from build123d import *

# Parameters (mm, degrees)
BOSS_EXTRUDE1_DEPTH = 25
FILLET1_R           = 5
SHELL1_T            = -2
SKETCH2_R           = 6.175
CUT_EXTRUDE2_DEPTH  = 25
CUT_EXTRUDE4_DEPTH  = 25
SKETCH4_R           = 1.25
SKETCH4_R_2         = 0.5
BOSS_EXTRUDE2_DEPTH = 7
SKETCH5_W           = 50.970389208
SKETCH5_H           = 16.037024898
CUT_EXTRUDE5_DEPTH  = 1.5


with BuildPart() as part:
    # Sketch1 → Boss-Extrude1 (new body)
    with BuildSketch(Plane.XY):
        with BuildLine():
            Line((-50, -62.5), (50, -62.5))
            ThreePointArc((50, -62.5), (53.535533906, -61.035533906), (55, -57.5))
            Line((55, -57.5), (55, 57.5))
            ThreePointArc((55, 57.5), (53.535533906, 61.035533906), (50, 62.5))
            Line((50, 62.5), (-50, 62.5))
            ThreePointArc((-50, 62.5), (-53.535533906, 61.035533906), (-55, 57.5))
            Line((-55, 57.5), (-55, -57.5))
            ThreePointArc((-55, -57.5), (-53.535533906, -61.035533906), (-50, -62.5))
        make_face()
    extrude(amount=BOSS_EXTRUDE1_DEPTH)

    # Fillet1
    fillet1_edges = [part.edges().sort_by_distance(p)[0] for p in [
        (53.535533906, -61.035533906, 25),
        (55, 0, 25),
        (53.535533906, 61.035533906, 25),
        (0, 62.5, 25),
        (-53.535533906, 61.035533906, 25),
        (-55, 0, 25),
        (-53.535533906, -61.035533906, 25),
        (0, -62.5, 25),
    ]]
    fillet(fillet1_edges, radius=FILLET1_R)

    # Shell1
    shell1_openings = [part.faces().sort_by_distance(p)[0] for p in [
        (0, 0, 0),
    ]]
    offset(amount=SHELL1_T, openings=shell1_openings, kind=Kind.INTERSECTION)

    # Sketch2 → Cut-Extrude2 (cut)
    with BuildSketch(Plane.XY.offset(25)):
        with Locations((-37.5, -45)):
            Circle(SKETCH2_R)
        with Locations((-12.5, -45)):
            Circle(SKETCH2_R)
        with Locations((12.5, -45)):
            Circle(SKETCH2_R)
        with Locations((37.5, -45)):
            Circle(SKETCH2_R)
        with Locations((-37.5, -23)):
            Circle(SKETCH2_R)
        with Locations((-12.5, -23)):
            Circle(SKETCH2_R)
        with Locations((12.5, -23)):
            Circle(SKETCH2_R)
        with Locations((37.5, -23)):
            Circle(SKETCH2_R)
        with Locations((-37.5, -1)):
            Circle(SKETCH2_R)
        with Locations((-12.5, -1)):
            Circle(SKETCH2_R)
        with Locations((12.5, -1)):
            Circle(SKETCH2_R)
        with Locations((37.5, -1)):
            Circle(SKETCH2_R)
        with Locations((-37.5, 21)):
            Circle(SKETCH2_R)
        with Locations((-12.5, 21)):
            Circle(SKETCH2_R)
        with Locations((12.5, 21)):
            Circle(SKETCH2_R)
        with Locations((37.5, 21)):
            Circle(SKETCH2_R)
    extrude(amount=-CUT_EXTRUDE2_DEPTH, mode=Mode.SUBTRACT)

    # Sketch3 → Cut-Extrude4 (cut)
    with BuildSketch(Plane.ZY.offset(55)):
        with BuildLine():
            Line((14.181299903, 43.9), (16.681299903, 42.5))
            ThreePointArc((16.681299903, 42.5), (17.034853293, 42.646446609), (17.181299903, 43))
            Line((17.181299903, 43), (17.181299903, 50))
            ThreePointArc((17.181299903, 50), (17.034853293, 50.353553391), (16.681299903, 50.5))
            Line((16.681299903, 50.5), (14.181299903, 49.1))
            Line((14.181299903, 49.1), (14.181299903, 43.9))
        make_face()
    extrude(amount=-CUT_EXTRUDE4_DEPTH, mode=Mode.SUBTRACT)

    # Sketch4 → Boss-Extrude2 (add)
    # profile 1 of 4: a face of its own
    with BuildSketch(Plane(origin=(0, 0, 17.181299903), x_dir=(-1, 0, 0), z_dir=(0, 0, -1))):
        with Locations((50.75, 40.469217889)):
            Circle(SKETCH4_R)
        with Locations((50.75, 40.469217889)):
            Circle(SKETCH4_R_2, mode=Mode.SUBTRACT)
    # profile 2 of 4: a face of its own
    with BuildSketch(Plane(origin=(0, 0, 17.181299903), x_dir=(-1, 0, 0), z_dir=(0, 0, -1))):
        with Locations((50.75, 52.469217889)):
            Circle(SKETCH4_R)
        with Locations((50.75, 52.469217889)):
            Circle(SKETCH4_R_2, mode=Mode.SUBTRACT)
    # profile 3 of 4: a face of its own
    with BuildSketch(Plane(origin=(0, 0, 17.181299903), x_dir=(-1, 0, 0), z_dir=(0, 0, -1))):
        with Locations((4.25, 52.469217889)):
            Circle(SKETCH4_R)
        with Locations((4.25, 52.469217889)):
            Circle(SKETCH4_R_2, mode=Mode.SUBTRACT)
    # profile 4 of 4: a face of its own
    with BuildSketch(Plane(origin=(0, 0, 17.181299903), x_dir=(-1, 0, 0), z_dir=(0, 0, -1))):
        with Locations((4.25, 40.469217889)):
            Circle(SKETCH4_R)
        with Locations((4.25, 40.469217889)):
            Circle(SKETCH4_R_2, mode=Mode.SUBTRACT)
    extrude(amount=-BOSS_EXTRUDE2_DEPTH)

    # Sketch5 → Cut-Extrude5 (cut)
    with BuildSketch(Plane(origin=(0, 0, 17.181299903), x_dir=(-1, 0, 0), z_dir=(0, 0, -1))):
        with Locations((26.773560326, 46.339549131)):
            Rectangle(SKETCH5_W, SKETCH5_H)
    extrude(amount=-CUT_EXTRUDE5_DEPTH, mode=Mode.SUBTRACT)


solid = part.part
Build history of the part. All positions in model axes, mm. A direction names the side the tool comes from. Round coordinates to 2 decimals unless told otherwise and drop trailing zeros. Write each loop counter-clockwise with the first axis right and the second up, starting at its lowest first coordinate (ties: lowest second). Pieces come first, ordered by that corner, then holes. Notation, with made-up numbers: M 2,19.5 L 55,19.5 A25 ccw 55,54.5 Z; hole C 85.25,54 d4. An arc over 180 degrees is marked long. Answer as a JSON object with one key per item and string values. Group by question number.
(1) Cut at B-B (y = -45). Give the cut face in (x, z) (3 decimals).
(2) Mould opens along Y. For faces 1 (the flat face through (-1, 1, 23)), 2 (the flat face through (-1, -62.5, 10)), 3 (the cylindrical face through (53.57, 61, 9.86)), 4 (the cylindrical face through (-43.67, -22.73, 24.01)) say: pulls with the +Y half, pulls with the -Y half, needs draft (parallel to the pull), parting line crosses it, or undercut.
(3) Cut at A-A (x = 37.5). Give the cut face in (y, z) (3 decimals), and give its area (3 significant figures).
(4) Which spindle directions (+Z, -Z, +X, -X, +Y, -Y) get a long thin tool onto all of the face, cutting with end or side? Do faces 5 (the flat face through (-53.2, 0.3, 0)), 6 (the flat face through (1, 60.5, 10)). Say none if no direction does.
(5) Drill centre lines: L1, parallel to X at y = 19.5, z = 6.25; L2, parallel to Y at x = -39.5, z = 7.5; L3, parallel to Y at x = -50.75, z = 21.2. Where is each one in solid material? Low to high.
(6) Flat gauge pins, fed straight in: pin 1 (1.1 mm diameter, centred on x = -4, y = 40.5, fed in from -Z); pin 2 (11 mm diameter, centred on x = -37.5, y = -45, fed in from +Z); pin 3 (14 mm diameter, centred on x = 12.5, y = -23, fed in from -Z); pin 4 (16 mm diameter, centred on x = 12.5, y = -1, fed in from +Z). Where does each tip first touch, or does it go through?
(7) Cut at C-C (z = 8.75). Give the cut face in (x, y).
Responses:
{
 "1": {"outline": "M -55,0 L -53,0 L -53,20 A3 cw -50,23 L -43.675,23 L -43.675,25 L -50,25 A5 ccw -55,20 Z; M -31.325,23 L -18.675,23 L -18.675,25 L -31.325,25 Z; M -6.325,23 L 6.325,23 L 6.325,25 L -6.325,25 Z; M 18.675,23 L 31.325,23 L 31.325,25 L 18.675,25 Z; M 43.675,23 L 50,23 A3 cw 53,20 L 53,0 L 55,0 L 55,20 A5 ccw 50,25 L 43.675,25 Z"},
 "2": {"face 1": "undercut", "face 2": "pulls with the -Y half", "face 3": "pulls with the +Y half", "face 4": "undercut"},
 "3": {"outline": "M -62.5,0 L -60.5,0 L -60.5,20 A3 cw -57.5,23 L -51.175,23 L -51.175,25 L -57.5,25 A5 ccw -62.5,20 Z; M -38.825,23 L -29.175,23 L -29.175,25 L -38.825,25 Z; M -16.825,23 L -7.175,23 L -7.175,25 L -16.825,25 Z; M 5.175,23 L 14.825,23 L 14.825,25 L 5.175,25 Z; M 27.175,23 L 57.5,23 A3 cw 60.5,20 L 60.5,0 L 62.5,0 L 62.5,20 A5 ccw 57.5,25 L 27.175,25 Z", "area": "236 mm2"},
 "4": {"face 5": "-Z, +X, -X, +Y, -Y", "face 6": "-Z"},
 "5": {"L1": "x = -55 to -53, 53 to 55", "L2": "y = -62.5 to -60.5, 60.5 to 62.5", "L3": "y = -62.3 to -60.15, 39.22 to 39.97, 40.97 to 41.72, 51.22 to 51.97, 52.97 to 53.72, 60.15 to 62.3"},
 "6": {"pin 1": "stops at z = 18.68", "pin 2": "passes through", "pin 3": "stops at z = 23", "pin 4": "stops at z = 25"},
 "7": {"outline": "M -55,-57.5 A5 ccw -50,-62.5 L 50,-62.5 A5 ccw 55,-57.5 L 55,57.5 A5 ccw 50,62.5 L -50,62.5 A5 ccw -55,57.5 Z; hole M -53,-57.5 A3 ccw -50,-60.5 L 50,-60.5 A3 ccw 53,-57.5 L 53,57.5 A3 ccw 50,60.5 L -50,60.5 A3 ccw -53,57.5 Z"}
}
